from build123d import *

# Parameters (mm, degrees)
BOSS_EXTRUDE1_DEPTH = 10
SKETCH2_W           = 90
SKETCH2_H           = 40
CUT_EXTRUDE1_DEPTH  = 10
SKETCH2_3_W         = 3
SKETCH2_3_H         = 3
SKETCH2_3_W_2       = 6
SKETCH2_3_H_2       = 6
CUT_EXTRUDE2_DEPTH  = 6
CHAMFER2_SIZE       = 5
CHAMFER2_SIZE_2     = 10.028448541
CHAMFER3_SIZE2      = 4.999988835
CHAMFER3_SIZE       = 10


# Some blends are built 0.0001 mm under size
with BuildPart() as part:
    # Sketch1 → Boss-Extrude1 (new body)
    with BuildSketch(Plane(origin=(0, 0, 0), x_dir=(1, 0, 0), z_dir=(0, 1, 0))):
        Polygon((-60, 50), (-60, -2.5), (-60, -50), (0, -50), (60, -50), (60, 50), (0, 50), align=None)
    extrude(amount=-BOSS_EXTRUDE1_DEPTH)

    # Sketch2 → Cut-Extrude1 (cut)
    with BuildSketch(Plane.XZ.offset(10)):
        with Locations((0, 25)):
            Rectangle(SKETCH2_W, SKETCH2_H)
    extrude(amount=-CUT_EXTRUDE1_DEPTH, mode=Mode.SUBTRACT)

    # Sketch2<3> → Cut-Extrude2 (cut)
    with BuildSketch(Plane.XZ.offset(10)):
        with Locations((47.5, 47.5)):
            Rectangle(SKETCH2_3_W, SKETCH2_3_H)
        with Locations((-47.5, 2.5)):
            Rectangle(SKETCH2_3_W, SKETCH2_3_H)
        with Locations((47.5, 2.5)):
            Rectangle(SKETCH2_3_W, SKETCH2_3_H)
        with Locations((45, -25)):
            Rectangle(SKETCH2_3_W_2, SKETCH2_3_H_2)
        with Locations((-47.5, 47.5)):
            Rectangle(SKETCH2_3_W, SKETCH2_3_H)
        with Locations((-45, -25)):
            Rectangle(SKETCH2_3_W_2, SKETCH2_3_H_2)
    extrude(amount=-CUT_EXTRUDE2_DEPTH, mode=Mode.SUBTRACT)

    # Chamfer2
    # the kernel refuses this chamfer: 10.028448541, 5 mm, written as the material it takes off along each edge
    with BuildSketch(Plane(origin=(-45, 0, 5), x_dir=(-0.9976061957759285, 0.06915112543899754, 0), z_dir=(0, 0, 1))) as chamfer2_piece_1:
        Polygon((CHAMFER2_SIZE * 0.997606195776, CHAMFER2_SIZE * 0.069151125439), (-CHAMFER2_SIZE_2 * 0.069151125441, CHAMFER2_SIZE_2 * 0.997606195805), (0, 0), align=None)
    extrude(amount=40, mode=Mode.SUBTRACT)

    # Chamfer3
    chamfer3_edges = [part.edges().sort_by_distance(p)[0] for p in [
        (45, 0, 25),
    ]]
    chamfer3_side = [part.faces().sort_by_distance(p)[0] for p in [
        (45, -0.099999777, 25),
    ]]
    chamfer(chamfer3_edges, length=CHAMFER3_SIZE - 0.0001, length2=CHAMFER3_SIZE2 - 0.0001, reference=chamfer3_side[0])  # a hair under: the kernel refuses the full size


solid = part.part
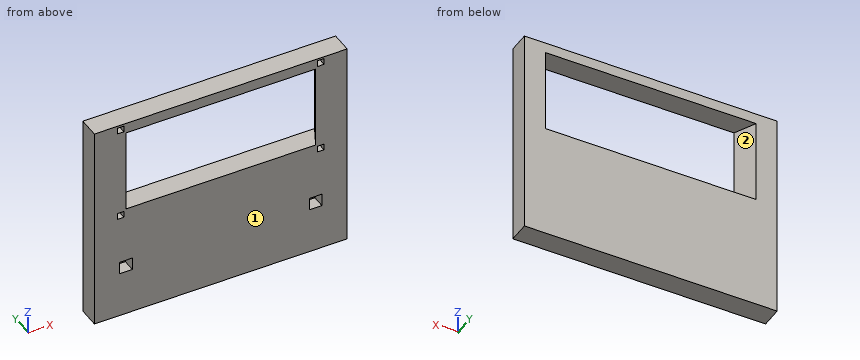
Input: part model. Units: mm. Frame: model coordinates. Face numbers are marked on the shaded views. Coordinates: 2 decimals unless noted, no trailing zeros. Write each loop counter-clockwise with the first axis right and the second up, starting at its lowest first coordinate (ties: lowest second). Pieces come first, ordered by that corner, then holes. Notation, with made-up numbers: M -19.75,-16 L -2.75,-16 A15 cw -2.75,-4 Z; hole C 89,16.25 d7. An arc over 180 degrees is marked long. Answer as a JSON object with one key per item and string values. Group by question number.
(1) Section D-D on y = -1.5. Output: boundary loops of the cut face in (x, z).
(2) Contact query for a flat-ended pin moving along its axis: P1, Ø1.5, axis at x = -47, z = 47, coming from the -Y side. Output: stop coordinate, or through.
(3) Ray query, line 1 along Z through (x, y) = (32, -8.25); line 2 along X through (y, z) = (-8, 11.5); line 3 along X through (y, z) = (-1.25, 6.5). Return the intervals inside material, ascending. Write a range as [from, to].
(4) Section B-B on x = -31.5. Output: boundary loops of the cut face in (y, z).
(5) Mould query, pull axis Z, two halves, no side actions, for the marked faces 1 and 2. Classes: pulls with the +Z half, pulls with the -Z half, needs draft (parallel to the pull), parting line crosses it, or undercut.
(6) Section C-C on y = -7.25. Give the number of separate pieces and of enclosed holes in the cut face, plus the area to 3 significant figures.
Result set:
{
 "1": {"outline": "M -60,-50 L 60,-50 L 60,50 L -60,50 Z; hole M -49.25,5 L 49.25,5 L 49.25,45 L -49.25,45 Z"},
 "2": {"P1": "stops at y = -4"},
 "3": {"line 1": "z = [-50, 5], [45, 50]", "line 2": "x = [-60, -46.01], [46, 60]", "line 3": "x = [-60, -49.38], [49.37, 60]"},
 "4": {"outline": "M -10,-50 L 0,-50 L 0,5 L -10,5 Z; M -10,45 L 0,45 L 0,50 L -10,50 Z"},
 "5": {"face 1": "needs draft", "face 2": "undercut"},
 "6": {"separate pieces": "1", "enclosed holes": "7", "area": "8,180 mm2"}
}
